Verification items for the finished model (mm, model axes). A direction names the side the tool comes from. Give positions to 0.01 mm unless a question says otherwise; leave off trailing zeros. Write each loop counter-clockwise with the first axis right and the second up, starting at its lowest first coordinate (ties: lowest second). Pieces come first, ordered by that corner, then holes. Notation, with made-up numbers: (-6, 49.5) - (45, 49.5) arc R28 cw to (45, 73.5) - close; hole circle Ø6 at (-5.5, 46.25). An arc over 180 degrees is marked (long way). Put each result on its own line as item: value.
from build123d import *

# Parameters (mm, degrees)
SKETCH1_R           = 35
SKETCH1_R_2         = 20
BOSS_EXTRUDE1_DEPTH = 75


with BuildPart() as part:
    # Sketch1 → Boss-Extrude1 (new body)
    # profile 1 of 2: a face of its own
    with BuildSketch(Plane.XY):
        Circle(SKETCH1_R)
        Circle(SKETCH1_R_2, mode=Mode.SUBTRACT)
    # profile 2 of 2: a face of its own
    with BuildSketch(Plane.XY):
        with BuildLine():
            ThreePointArc((-34.186985828, 7.5), (-32.736987087, 12.381020816), (-30.594117082, 17))
            Line((-30.594117082, 17), (-55, 17))
            ThreePointArc((-55, 17), (-72, 0), (-55, -17))
            Line((-55, -17), (-30.594117082, -17))
            ThreePointArc((-30.594117082, -17), (-32.736987087, -12.381020816), (-34.186985828, -7.5))
            Line((-34.186985828, -7.5), (-55, -7.5))
            ThreePointArc((-55, -7.5), (-62.5, 0), (-55, 7.5))
            Line((-55, 7.5), (-34.186985828, 7.5))
        make_face()
    extrude(amount=BOSS_EXTRUDE1_DEPTH)


solid = part.part
Q1. Release check for a two-part mould opening along X. For faces 5 (the face through (-44, -7.5, 37)), 6 (the face through (-19, -7, 75)), 7 (the face through (-72, 0, 37)) record: released by +X, released by -X, zero draft, split by the parting line, or undercut.
Answers follow:
face 5: undercut
face 6: zero draft
face 7: released by -X
Q2. Set-up check for faces 1 (the face through (-45, 7.5, 37)), 2 (the face through (-43, -17, 37)), 3 (the face through (-19, -7, 0)), 4 (the face through (-43, 17, 37)): record each of +Z, -Z, +X, -X, +Y, -Y from which the full face is reachable in a straight line by a thin tool's end or side.
Answers follow:
face 1: +Z, -Z
face 2: +Z, -Z, -X, -Y
face 3: -Z, +X, -X, +Y, -Y
face 4: +Z, -Z, -X, +Y
Q3. Section check D-D, the plane x = -45. Record the cut outline in (y, z).
Answers follow:
outline: (-17, 0) - (-7.5, 0) - (-7.5, 75) - (-17, 75) - close; (7.5, 0) - (17, 0) - (17, 75) - (7.5, 75) - close
Q4. Section check B-B, the plane y = 0. Record the cut outline in (x, z), plus the area to 3 significant figures.
Answers follow:
outline: (-72, 0) - (-62.5, 0) - (-62.5, 75) - (-72, 75) - close; (-35, 0) - (-20, 0) - (-20, 75) - (-35, 75) - close; (20, 0) - (35, 0) - (35, 75) - (20, 75) - close
area: 2,960 mm2
Q5. Go/stop test with flat-tipped pins: pin 1 Ø1.5 at (x, z) = (-23, 9.5) entering from -Y; pin 2 Ø3 at (x, z) = (-55.5, 61.5) entering from +Y; pin 3 Ø6 at (x, z) = (19.5, 24.5) entering from -Y. Record where each tip stops, or that it passes through.
Answers follow:
pin 1: stops at y = -27.02
pin 2: stops at y = 17
pin 3: stops at y = -30.87
Q6. Section check A-A, the plane x = 0. Record the cut outline in (y, z), plus the area to 3 significant figures.
Answers follow:
outline: (-35, 0) - (-20, 0) - (-20, 75) - (-35, 75) - close; (20, 0) - (35, 0) - (35, 75) - (20, 75) - close
area: 2,250 mm2
Q7. Section check C-C, the plane z = 67.5. Record the cut outline in (x, y).
Answers follow:
outline: (-55, -17) - (-30.59, -17) arc R35 ccw (long way) to (-30.59, 17) - (-55, 17) arc R17 ccw to start; hole (-55, -7.5) - (-34.19, -7.5) arc R35 cw to (-34.19, 7.5) - (-55, 7.5) arc R7.5 ccw to start; hole circle Ø40 at (0, 0)
Q8. Scan lines: line 1 along Y through (x, z) = (-35.5, 25.5); line 2 along Y through (x, z) = (0, 29); line 3 along X through (y, z) = (5.5, 17.5). Record each from-to range of solid material in increasing order.
Answers follow:
line 1: y = -17 to -7.5, 7.5 to 17
line 2: y = -35 to -20, 20 to 35
line 3: x = -71.09 to -60.1, -34.57 to -19.23, 19.23 to 34.57
